Autodesk Inventor part; units mm, degrees
ref_plane "YZ Plane" through (0, 0, 0) normal (1, 0, 0) x (0, 1, 0)
ref_plane "XZ Plane" through (0, 0, 0) normal (0, 1, 0) x (-1, 0, 0)
ref_plane "XY Plane" through (0, 0, 0) normal (0, 0, 1) x (1, 0, 0)
sketch "Boceto1" plane through (0, 0, 0) normal (0, 1, 0) x (-1, 0, 0)
  line L0 (0, 0) -> (0, -55)
  line L1 (0, -55) -> (0, 55)
  line L2 (0, 55) -> (105, 55)
  line L3 (105, 55) -> (105, -55)
  line L4 (105, -55) -> (0, -55)
  dimension "d0" = 55
  dimension "d1" = 110
  dimension "d2" = 105
  dimension "d3" = 110
extrude "Extrusión1" add sketch "Boceto1" along normal blind 30
sketch "Boceto2" plane through (0, 0, 55) normal (1, 0, 0) x (0, 0, -1)
  line L0 (0, 0) -> (0, 30)
  line L1 (0, 0) -> (0, 5)
  line L2 (0, 5) -> (110, 5)
  line L3 (110, 0) -> (110, 30)
  line L4 (110, 30) -> (0, 30)
  line L5 (0, 30) -> (0, 25)
  line L6 (0, 25) -> (110, 25)
  line L7 (0, 30) -> (5, 30)
  line L8 (5, 30) -> (5, 0)
  line L9 (110, 0) -> (0, 0)
  line L10 (110, 30) -> (105, 30)
  line L11 (105, 30) -> (105, 0)
  point P0 (55, 0)
  point P1 (105, 5)
  point P2 (105, 25)
  point P3 (5, 25)
  point P4 (5, 5)
  dimension "d6" = 5
  dimension "d7" = 5
  dimension "d9" = 110
  dimension "d10" = 5
  dimension "d11" = 5
extrude "Extrusión2" cut sketch "Boceto2" against normal blind 100 contours L8 L6 L11 L2
sketch "Boceto3" plane through (0, 0, 0) normal (0, -1, 0) x (1, 0, 0)
  line L0 (0, 55.0451) -> (0, 45.0451)
  line L1 (0, -50) -> (0, 50)
  line L2 (0, 45.0451) -> (-10, 45.0451)
  line L3 (-105, 55) -> (0, 55)
  line L4 (0, 55) -> (-10, 55)
  line L5 (-10, 45.0451) -> (-10, 55)
  line L6 (0, 0) -> (-105, 0)
  line L7 (-105, -55) -> (-105, 55)
  line L8 (-105, 55) -> (-105, 45)
  line L9 (-105, 45) -> (-95, 45)
  line L10 (-95, 45) -> (-95, 55)
  line L11 (-105, 55) -> (-95, 55)
  line L12 (0, -55.0451) -> (0, -45.0451)
  line L13 (0, -45.0451) -> (-10, -45.0451)
  line L14 (-105, -55) -> (0, -55)
  line L15 (-10, -45.0451) -> (-10, -55)
  line L16 (-105, 55) -> (-105, -55)
  line L17 (-105, -45) -> (-95, -45)
  line L18 (-95, -45) -> (-95, -55)
  dimension "d14" = 10
  dimension "d15" = 10
  dimension "d16" = 10
  dimension "d17" = 10
extrude "Extrusión3" add sketch "Boceto3" along normal blind 100 contours L0 L2 L5 L3 | L10 L9 L7 L3 | L1 L12 L14 L15 L13 | L17 L18 L14 L7
fillet "Empalme1" radius 2 5 edges at (-52.5, 30, 55) (-52.5, 30, -55) (-105, 30, 0) (0, 30, 0) (0, 0, 0)
properties part number "Base_carga"
Geometry check sheet. Reference: the model listing, model coordinates, mm. A direction names the side the tool comes from. Round coordinates to 2 decimals unless told otherwise and drop trailing zeros. Order: outer loops, then holes, each group sorted by start corner. A loop starts at its lowest first (then second) coordinate and runs counter-clockwise, first axis right, second up. Notation, with made-up numbers: M -24,25.25 L -19,25.25 A36 cw -19,59.25 Z; hole C 20,-12.75 d8. An arc over 180 degrees is marked long. Write item = value, one per line.
Q1. Set-up check for faces 4 (the flat face through (-49, 15, -50)), 5 (the flat face through (-10, -49, -50)): record each of +Z, -Z, +X, -X, +Y, -Y from which the full face is reachable in a straight line by a thin tool's end or side.
Answer block:
face_4 = +X
face_5 = +Z, -Z, -Y
Q2. Section check B-B (y = -20). Enter the section's corners in (x, z).
Answer block:
outline = M -105,-55 L -95,-55 L -95,-45 L -105,-45 Z; M -105,45 L -95,45 L -95,55 L -105,55 Z; M -10,-55 L 0,-55 L 0,-45.05 L -10,-45.05 Z; M -10,45.05 L 0,45.05 L 0,55 L -10,55 Z
Q3. Section check A-A (x = -93). Enter the section's corners in (y, z), plus the area to 3 significant figures.
Answer block:
outline = M 0,-55 L 28,-55 A2 ccw 30,-53 L 30,53 A2 ccw 28,55 L 0,55 Z; hole M 5,-50 L 25,-50 L 25,50 L 5,50 Z
area = 1,300 mm^2
Q4. Section check C-C (y = 11). Enter the section's corners in (x, z), plus the area to 3 significant figures.
Answer block:
outline = M -105,-55 L 0,-55 L 0,-50 L -100,-50 L -100,50 L 0,50 L 0,55 L -105,55 Z
area = 1,550 mm^2
Q5. Scan lines: line 1 (Y direction, x = -69, z = -40.5); line 2 (X direction, y = -70.5, z = -50); line 3 (Z direction, x = -73, y = 21.5). Record each from-to range of solid material in increasing order.
Answer block:
line_1 = 0 to 5, 25 to 30
line_2 = -105 to -95, -10 to 0
line_3 = -55 to -50, 50 to 55
Q6. Release check for a two-part mould opening along X. For faces 1 (the flat face through (-100, 15, 1)), 2 (the flat face through (-95, -49, -50)), 3 (the flat face through (-49, 15, 50)) record: released by +X, released by -X, zero draft, split by the parting line, or undercut.
Answer block:
face_1 = released by +X
face_2 = undercut
face_3 = zero draft
Q7. Section check D-D (z = -21.5). Enter the section's corners in (x, y), plus the area to 3 significant figures.
Answer block:
outline = M -105,0 L -2,0 A2 ccw 0,2 L 0,5 L -100,5 L -100,25 L 0,25 L 0,28 A2 ccw -2,30 L -103,30 A2 ccw -105,28 Z
area = 1,150 mm^2
Q8. Depth check by flat-ended pin: pin 1 Ø4 at (x, z) = (-27, -41) entering from -Y; pin 2 Ø10 at (y, z) = (19, 23.5) entering from +X. Enter the tip coordinate at first touch or a pass-through.
Answer block:
pin_1 = 0
pin_2 = -100
